Design review of the part shown in the three views and the two pictorial views. Dimensions are in mm from the part's minimum x, y and z. Coordinates: 2 decimals unless noted, no trailing zeros. Loops run counter-clockwise (first coordinate to the right, second up) from the corner with the lowest first, then second, coordinate; pieces in that order, holes last. Notation, with made-up numbers: (14.5, -4.5) -> (73.5, -4.5) arc R24 cw to (73.5, 22.5) -> close; hole circle Ø2 at (16.25, -36.5). An arc over 180 degrees is marked (long way). Answer in a Markdown table with one row per item.
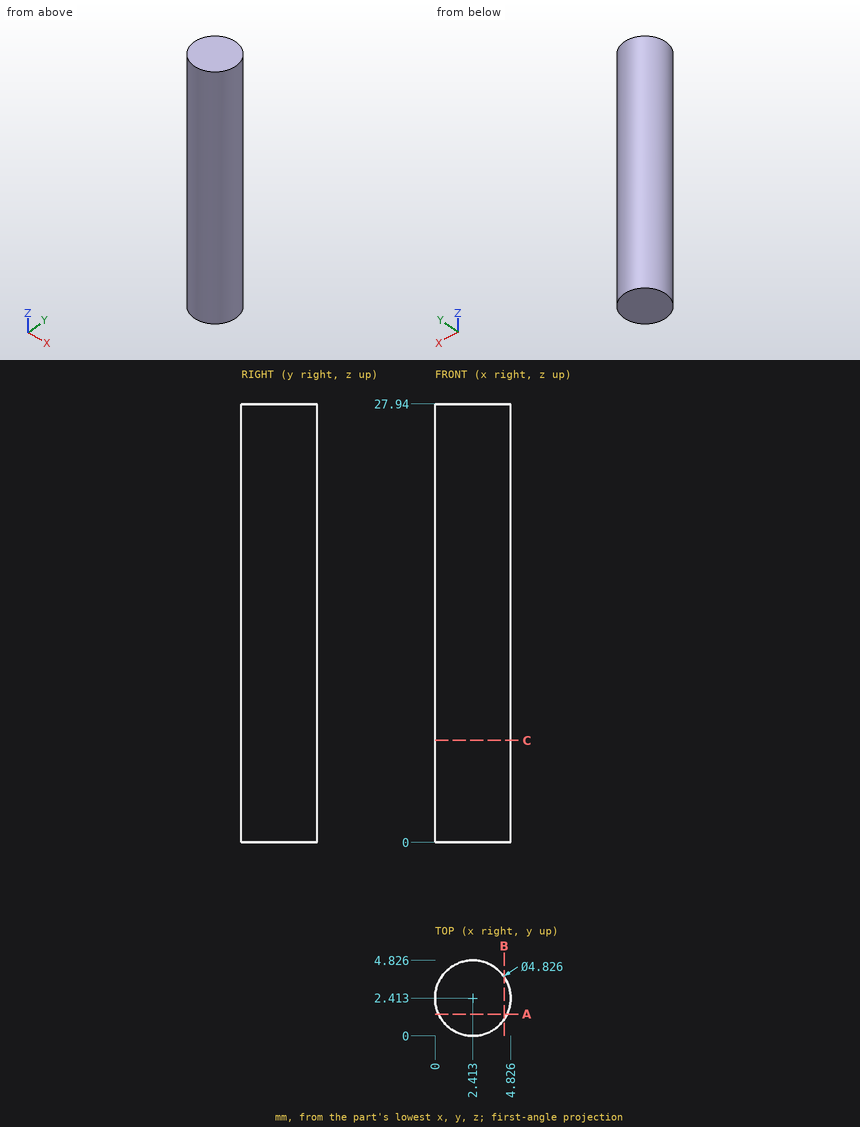
Item 1: For L1, parallel to X at y = 0.45, z = 26.25; L2, parallel to Y at x = 2, z = 6.5; L3, parallel to Y at x = 0.75, z = 10.75, list the stretches that pass through material, from the lowest coordinate up.
Worked answers:
| item | result |
|---|---|
| L1 | 1.01 to 3.82 |
| L2 | 0.04 to 4.79 |
| L3 | 0.66 to 4.16 |
Item 2: Insertion check: pin 1 (2 mm diameter, centred on x = 0.5, z = 12, fed in from +Y). The pin has a flat end and moves straight along its axis. Give the tip position at first contact, or say it passes through.
Worked answers:
| item | result |
|---|---|
| pin 1 | y = 4.65 |
Item 3: Take a section at A-A, the plane y = 1.4. State the section outline as (x, z) points.
Worked answers:
| item | result |
|---|---|
| outline | (0.22, 0) -> (4.6, 0) -> (4.6, 27.94) -> (0.22, 27.94) -> close |
Item 4: Take a section at B-B, the plane x = 4.4. State the section outline as (y, z) points, and give its area (3 significant figures).
Worked answers:
| item | result |
|---|---|
| outline | (1.04, 0) -> (3.78, 0) -> (3.78, 27.94) -> (1.04, 27.94) -> close |
| area | 76.5 mm² |
Item 5: Take a section at C-C, the plane z = 6.5. State the section outline as (x, y) points.
Worked answers:
| item | result |
|---|---|
| outline | circle Ø4.83 at (2.41, 2.41) |
